The model under review builds one solid part; all positions refer to its coordinate system, in mm. Face numbers are marked on the shaded views. Coordinates: 2 decimals unless noted, no trailing zeros. Order: outer loops, then holes, each group sorted by start corner. A loop starts at its lowest first (then second) coordinate and runs counter-clockwise, first axis right, second up. Notation, with made-up numbers: (13.5, -39) -> (42.5, -39) arc R24 cw to (42.5, -17) -> close; hole circle Ø5 at (-10.75, 58). An arc over 180 degrees is marked (long way). Use one line per item in the form item = value.
from build123d import *

# Parameters (mm, degrees)
F0_R     = 47.5
F1_DEPTH = 25
F2_R     = 25
F3_DEPTH = 15
F4_R     = 10


with BuildPart() as f1:
    # F0 (on Top) → F1 (new body)
    with BuildSketch(Plane.XY):
        Circle(F0_R)
    extrude(amount=F1_DEPTH)

    # F2 (on face) → F3 (cut)
    with BuildSketch(Plane.XY.offset(25)):
        Circle(F2_R)
    extrude(amount=-F3_DEPTH, mode=Mode.SUBTRACT)

    # F4
    f4_edges = [f1.edges().sort_by_distance(p)[0] for p in [
        (-47.5, 0, 25),
        (-25, 0, 25),
    ]]
    fillet(f4_edges, radius=F4_R)

    # F5 (on Front) → F6 (revolve, cut)
    with BuildSketch(Plane.XZ):
        with BuildLine():
            Line((-50.882176, -0.324849), (-47.5, 0))
            Line((-47.5, 0), (-47.5, 1.3))
            Line((-47.5, 1.3), (-45.5, 1.3))
            Line((-45.5, 1.3), (-47.322187, 13.587635))
            ThreePointArc((-47.322187, 13.587635), (-44.992555, 21.59772), (-37.400495, 25.054492))
            Line((-37.400495, 25.054492), (-37.400495, 26.943451))
            Line((-37.400495, 26.943451), (-49.502667, 21.701315))
            Line((-49.502667, 21.701315), (-50.882176, -0.324849))
        make_face()
    revolve(axis=Axis((0, 0, 17.452553), (0, 0, 1)), mode=Mode.SUBTRACT)


solid = f1.part
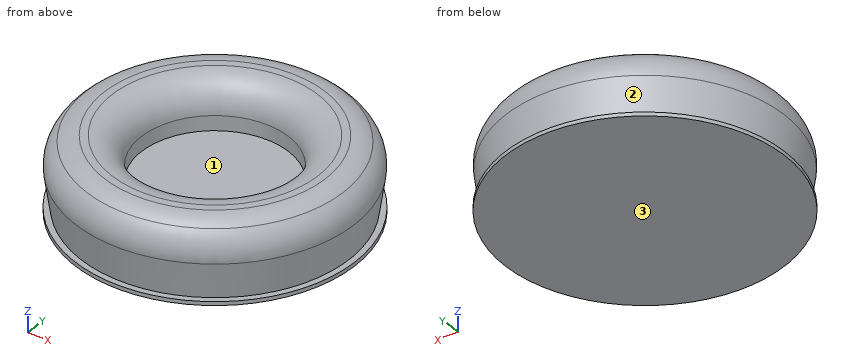
Item 1: We need section A-A (y = 0). Write out the cut boundary in (x, z).
Results found:
outline = (-47.5, 0) -> (47.5, 0) -> (47.5, 1.3) -> (45.5, 1.3) -> (47.32, 13.59) arc R10 ccw to (43.63, 22.9) arc R10 ccw to (37.5, 25) -> (35, 25) arc R10 ccw to (25, 15) -> (25, 10) -> (-25, 10) -> (-25, 15) arc R10 ccw to (-35, 25) -> (-37.5, 25) arc R10 ccw to (-43.63, 22.9) arc R10 ccw to (-47.32, 13.59) -> (-45.5, 1.3) -> (-47.5, 1.3) -> close
Item 2: Clearance check with flat-ended pins moving along their axes: pin 1 (12 mm diameter, centred on x = -29.5, z = 12, fed in from -Y); pin 2 (1 mm diameter, centred on y = 23.5, z = 13, fed in from +X); pin 3 (4 mm diameter, centred on x = 35, z = 20, fed in from -Y); pin 4 (1 mm diameter, centred on x = -2.5, y = 6, fed in from -Z). State where each tip first meets the part, or that it passes through.
Results found:
pin_1 = -40.95
pin_2 = 41.27
pin_3 = -32.66
pin_4 = 0
Item 3: To check wall thickness, follow L1, parallel to Z at x = 13, y = 20; L2, parallel to Y at x = 0, z = 12.85; L3, parallel to Y at x = 0, z = 12. State the ranges of each line that lie inside material, in increasing order. Write a range as from..to.
Results found:
L1 = 0..10
L2 = -47.21..-25, 25..47.21
L3 = -47.09..-25, 25..47.09
Item 4: We need section C-C (z = 3). Write out the cut boundary in (x, y), plus the area to 3 significant figures.
Results found:
outline = circle Ø91.5 at (0, 0)
area = 6,580 mm²
Item 5: Draft analysis for pull direction Y (two halves, no side actions). For the marked faces 1, 2 and 3, state which applies: released by +Y, released by -Y, zero draft, split by the parting line, or undercut.
Results found:
face_1 = undercut
face_2 = split by the parting line
face_3 = zero draft
